Geometry: final body of the model. Coordinates: model frame, mm. Face numbers are marked on the shaded views. A direction names the side the tool comes from. Coordinates: 2 decimals unless noted, no trailing zeros. Loops run counter-clockwise (first coordinate to the right, second up) from the corner with the lowest first, then second, coordinate; pieces in that order, holes last. Notation, with made-up numbers: (82, 82) - (114, 82) arc R18 cw to (114, 108) - close; hole circle Ø9 at (-9, 37). An arc over 180 degrees is marked (long way). Return JSON: item names as keys, results as strings.
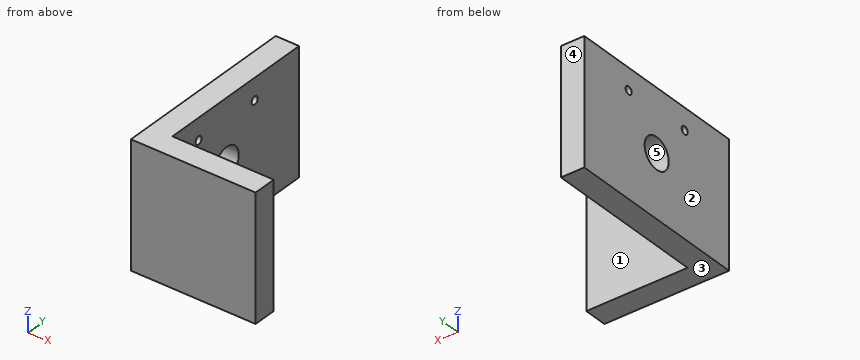
from build123d import *

# Parameters (mm, degrees)
BOSS_EXTRUDE1_DEPTH = 25.4
SKETCH3_R           = 6.35
CUT_EXTRUDE1_DEPTH  = 91.306287849
SKETCH4_R           = 1.5875
CUT_EXTRUDE2_DEPTH  = 91.306287849


with BuildPart() as part:
    # Sketch2 → Boss-Extrude1 (new, symmetric)
    with BuildSketch(Plane.XY):
        Polygon((0, 0), (0, 76.2), (9.525, 76.2), (9.525, 9.525), (50.8, 9.525), (50.8, 0), align=None)
    extrude(amount=BOSS_EXTRUDE1_DEPTH, both=True)

    # Sketch3 → Cut-Extrude1 (cut, through all)
    with BuildSketch(Plane(origin=(9.525, 0, 0), x_dir=(0, 0, -1), z_dir=(1, 0, 0))):
        with Locations(Location((0, 38.1, 0), (0, 0, 90))):
            Circle(SKETCH3_R)
    extrude(amount=-CUT_EXTRUDE1_DEPTH, mode=Mode.SUBTRACT)

    # Sketch4 → Cut-Extrude2 (cut, through all)
    with BuildSketch(Plane(origin=(9.525, 0, 0), x_dir=(0, 0, -1), z_dir=(1, 0, 0))):
        with Locations(Location((-16.621505447, 52.853853113, 0), (0, 0, 90))):
            Circle(SKETCH4_R)
        with Locations(Location((-16.621505447, 23.346146887, 0), (0, 0, 90))):
            Circle(SKETCH4_R)
    extrude(amount=-CUT_EXTRUDE2_DEPTH, mode=Mode.SUBTRACT)


solid = part.part
Item 1: Section query C-C, the plane z = -10. Return loops of the section in (x, y) (3 decimals).
Worked out:
{"outline": "(0, 0) - (50.8, 0) - (50.8, 9.525) - (9.525, 9.525) - (9.525, 76.2) - (0, 76.2) - close"}
Item 2: Section query D-D, the plane x = 35.5. Return loops of the section in (y, z) (3 decimals), and give its area (3 significant figures).
Worked out:
{"outline": "(0, -25.4) - (9.525, -25.4) - (9.525, 25.4) - (0, 25.4) - close", "area": "484 mm^2"}
Item 3: Reachability of the marked faces 1 and 2 from +Z, -Z, +X, -X, +Y, -Y: full face, straight path, thin tool, end or side. Return the list, or none.
Worked out:
{"face 1": "+Z, -Z, +X, +Y", "face 2": "+Z, -Z, -X, +Y, -Y"}
Item 4: Section query B-B, the plane y = 38.1. Return loops of the section in (x, z) (3 decimals).
Worked out:
{"outline": "(0, -25.4) - (9.525, -25.4) - (9.525, -6.35) - (0, -6.35) - close; (0, 6.35) - (9.525, 6.35) - (9.525, 25.4) - (0, 25.4) - close"}
Item 5: Section query A-A, the plane z = 0. Return loops of the section in (x, y) (3 decimals).
Worked out:
{"outline": "(0, 0) - (50.8, 0) - (50.8, 9.525) - (9.525, 9.525) - (9.525, 31.75) - (0, 31.75) - close; (0, 44.45) - (9.525, 44.45) - (9.525, 76.2) - (0, 76.2) - close"}
Item 6: First-contact query: pin 1 Ø10 at (y, z) = (38, 12.5) entering from +X (3 decimals); pin 2 Ø20.5 at (x, z) = (23, -12) entering from +Y (3 decimals). Flat tips, straight axial feed; report the tip coordinate or a pass-through.
Worked out:
{"pin 1": "x = 9.525", "pin 2": "y = 9.525"}
Item 7: Mould query, pull axis Y, two halves, no side actions, for the marked faces 3, 4 and 5. Classes: +Y half, -Y half, draft (parallel to the pull), parting line (faces both ways), or undercut.
Worked out:
{"face 3": "draft", "face 4": "+Y half", "face 5": "undercut"}
Item 8: Ray query, probe 1 along Z at (x, y) = (2, 38); probe 2 along X at (y, z) = (23, -12) (3 decimals). Return the intervals inside material, ascending. Write a range as from..to.
Worked out:
{"probe 1": "-25.4..-6.35, 6.35..25.4", "probe 2": "0..9.525"}
